Answer from the drawing. Dimensions are ordinates in mm from the lowest x, y and z of the part. A direction names the side the tool comes from. Give positions to 0.01 mm unless a question says otherwise; leave off trailing zeros. Write each loop counter-clockwise with the first axis right and the second up, starting at its lowest first coordinate (ties: lowest second). Pieces come first, ordered by that corner, then holes. Notation, with made-up numbers: M -24.5,31 L 3.5,31 A17 ccw 3.5,50 Z; hole C 56.5,61 d5. An arc over 180 degrees is marked long. Answer as a JSON object with one key per item and string values.
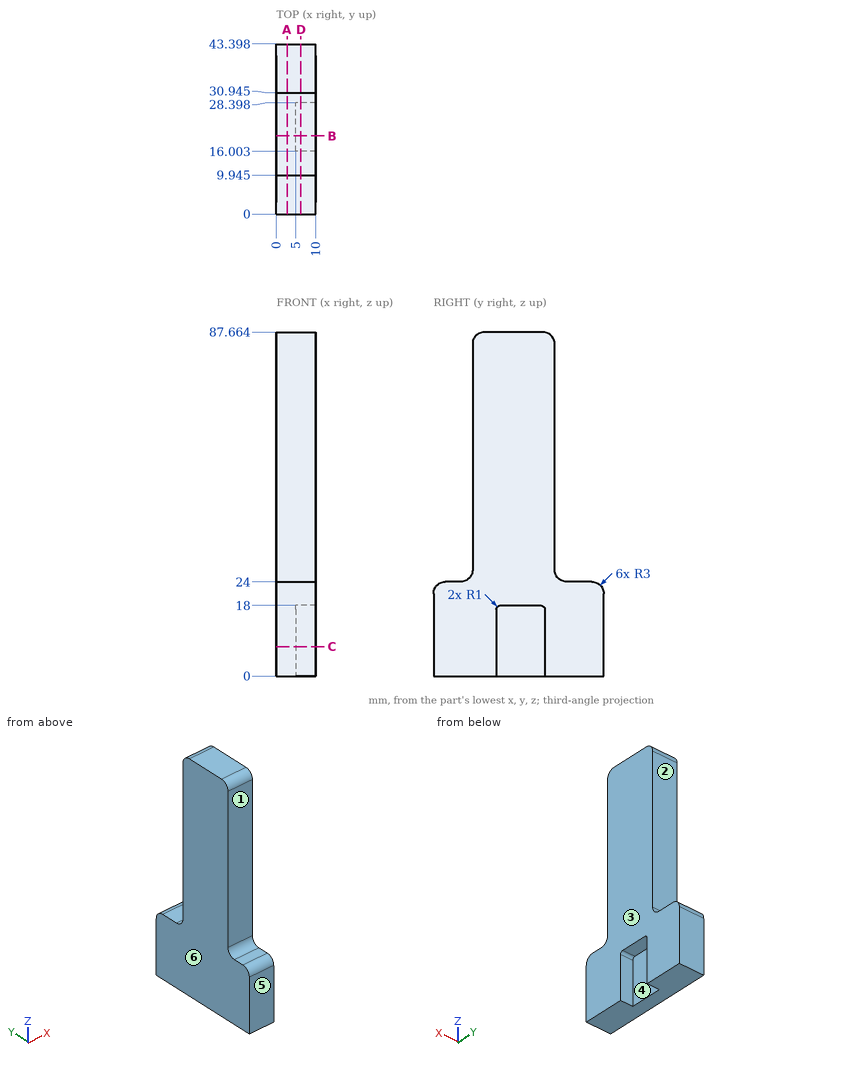
1. A cutting plane is placed at C-C, the plane z = 7.5. Give the vertices of the cut face in (x, y).
Verdict:
{"outline": "M 0,0 L 10,0 L 10,16 L 5,16 L 5,28.4 L 10,28.4 L 10,43.4 L 0,43.4 Z"}
2. The mould has two halves that part along Y. Classify the marked faces 4, 5 and 6: released by +Y, released by -Y, zero draft, split by the parting line, or undercut.
Verdict:
{"face 4": "undercut", "face 5": "released by -Y", "face 6": "zero draft"}
3. A cutting plane is placed at D-D, the plane x = 6.25. Give the vertices of the cut face in (y, z) (1 decimal), plus the area to 3 significant figures.
Verdict:
{"outline": "M 0,0 L 16,0 L 16,17 A1 cw 17,18 L 27.4,18 A1 cw 28.4,17 L 28.4,0 L 43.4,0 L 43.4,21 A3 ccw 40.4,24 L 33.9,24 A3 cw 30.9,27 L 30.9,84.7 A3 ccw 27.9,87.7 L 12.9,87.7 A3 ccw 9.9,84.7 L 9.9,27 A3 cw 6.9,24 L 3,24 A3 ccw 0,21 Z", "area": "2,150 mm2"}
4. A cutting plane is placed at A-A, the plane x = 2.75. Give the vertices of the cut face in (y, z) (1 decimal).
Verdict:
{"outline": "M 0,0 L 43.4,0 L 43.4,21 A3 ccw 40.4,24 L 33.9,24 A3 cw 30.9,27 L 30.9,84.7 A3 ccw 27.9,87.7 L 12.9,87.7 A3 ccw 9.9,84.7 L 9.9,27 A3 cw 6.9,24 L 3,24 A3 ccw 0,21 Z"}
5. For the marked faces 1, 2 and 3, determine the directions among +Z, -Z, +X, -X, +Y, -Y from which every point of the face is accessible in a straight line to the end or side of a thin tool.
Verdict:
{"face 1": "+Z, +X, -X, -Y", "face 2": "+Z, +X, -X, +Y", "face 3": "+Z, -Z, +X, +Y, -Y"}
6. Consider line 1 along Y through (x, z) = (5.75, 17); line 2 along Y through (x, z) = (8.5, 75) (1 decimal); line 3 along Z through (x, y) = (1.75, 35). Determine where each line is inside the solid, lowest interval first.
Verdict:
{"line 1": "y = 0 to 16, 28.4 to 43.4", "line 2": "y = 9.9 to 30.9", "line 3": "z = 0 to 24"}
7. A cutting plane is placed at B-B, the plane y = 20. Give the vertices of the cut face in (x, z).
Verdict:
{"outline": "M 0,0 L 5,0 L 5,18 L 10,18 L 10,87.66 L 0,87.66 Z"}
8. Flat-ended cylindrical pins translate along their axes: pin 1 (3 mm diameter, centred on x = 6.5, y = 36.5, fed in from +Z); pin 2 (5 mm diameter, centred on x = 6.5, z = 46.5, fed in from -Y) (1 decimal); pin 3 (1.5 mm diameter, centred on x = 8, y = 22, fed in from -Z). Find the tip coordinate at first contact, or state that the pin passes through.
Verdict:
{"pin 1": "stops at z = 24", "pin 2": "stops at y = 9.9", "pin 3": "stops at z = 18"}
